Work out the finished part from the listing and answer in its coordinate system (mm). A direction names the side the tool comes from. Round coordinates to 2 decimals unless told otherwise and drop trailing zeros. Write each loop counter-clockwise with the first axis right and the second up, starting at its lowest first coordinate (ties: lowest second). Pieces come first, ordered by that corner, then holes. Notation, with made-up numbers: M 11.5,29.25 L 56.5,29.25 A23 ccw 56.5,59.25 Z; hole C 54,29 d4. An arc over 180 degrees is marked long. Answer in a Markdown table with one row per item.
```python
from build123d import *

# Parameters (mm, degrees)
SKETCH1_R           = 2
SKETCH1_W           = 10
SKETCH1_H           = 28
SKETCH1_W_2         = 12
SKETCH1_H_2         = 48
BOSS_EXTRUDE1_DEPTH = 5
SKETCH1_3_R         = 3.5
BOSS_EXTRUDE2_DEPTH = 8


with BuildPart() as part:
    # Sketch1 → Boss-Extrude1 (new body)
    with BuildSketch(Plane(origin=(0, 0, 0), x_dir=(1, 0, 0), z_dir=(0, 1, 0))):
        with BuildLine():
            Line((0, -9), (0, 9))
            Line((0, 9), (6, 19))
            Line((6, 19), (14, 23.618802154))
            Line((14, 23.618802154), (22, 34))
            Line((22, 34), (22, 40))
            ThreePointArc((22, 40), (23.757359313, 44.242640687), (28, 46))
            Line((28, 46), (36, 46))
            ThreePointArc((36, 46), (40.242640687, 44.242640687), (42, 40))
            Line((42, 40), (42, 34))
            Line((42, 34), (57, 34))
            Line((57, 34), (67, 44))
            Line((67, 44), (87, 44))
            Line((87, 44), (87, 41))
            Line((87, 41), (69, 41))
            Line((69, 41), (69, 37))
            Line((69, 37), (97, 37))
            Line((97, 37), (97, 25))
            Line((97, 25), (87, 25))
            Line((87, 25), (87, 14))
            Line((87, 14), (82, 14))
            Line((82, 14), (82, -14))
            Line((82, -14), (87, -14))
            Line((87, -14), (87, -25))
            Line((87, -25), (97, -25))
            Line((97, -25), (97, -37))
            Line((97, -37), (69, -37))
            Line((69, -37), (69, -41))
            Line((69, -41), (87, -41))
            Line((87, -41), (87, -44))
            Line((87, -44), (67, -44))
            Line((67, -44), (57, -34))
            Line((57, -34), (42, -34))
            Line((42, -34), (42, -40))
            ThreePointArc((42, -40), (40.242640687, -44.242640687), (36, -46))
            Line((36, -46), (28, -46))
            ThreePointArc((28, -46), (23.757359313, -44.242640687), (22, -40))
            Line((22, -40), (22, -34))
            Line((22, -34), (14, -23.618802154))
            Line((14, -23.618802154), (6, -19))
            Line((6, -19), (0, -9))
        make_face()
        with Locations(Location((57, -27, 0), (0, 0, 270))):
            Circle(SKETCH1_R, mode=Mode.SUBTRACT)
        with Locations(Location((7, -10, 0), (0, 0, 270))):
            Circle(SKETCH1_R, mode=Mode.SUBTRACT)
        with Locations(Location((57, 27, 0), (0, 0, 270))):
            Circle(SKETCH1_R, mode=Mode.SUBTRACT)
        with Locations(Location((7, 10, 0), (0, 0, 270))):
            Circle(SKETCH1_R, mode=Mode.SUBTRACT)
        with Locations((66, 0)):
            Rectangle(SKETCH1_W, SKETCH1_H, mode=Mode.SUBTRACT)
        Polygon((14, 19), (23, 24), (23, -24), (14, -19), align=None, mode=Mode.SUBTRACT)
        with Locations((35, 0)):
            Rectangle(SKETCH1_W_2, SKETCH1_H_2, mode=Mode.SUBTRACT)
    extrude(amount=BOSS_EXTRUDE1_DEPTH)

    # Sketch1_3 → Boss-Extrude2 (add)
    with BuildSketch(Plane(origin=(0, 0, 0), x_dir=(1, 0, 0), z_dir=(0, 1, 0))):
        with Locations(Location((32, -40, 0), (0, 0, 270))):
            Circle(SKETCH1_3_R)
        with Locations(Location((32, 40, 0), (0, 0, 270))):
            Circle(SKETCH1_3_R)
    extrude(amount=BOSS_EXTRUDE2_DEPTH)


solid = part.part
```
1. The part is cut by section B-B (z = 17). Determine the outline of the cut face in (x, y).
Calculated:
| item | result |
|---|---|
| outline | M 4.8,0 L 14,0 L 14,5 L 4.8,5 Z; M 23,0 L 29,0 L 29,5 L 23,5 Z; M 41,0 L 87,0 L 87,5 L 41,5 Z |
2. Determine the mould class of faces 1 (the flat face through (84, 2, 14)), 2 (the flat face through (23, 2, 0)), 3 (the flat face through (87, 2, -20)) for opening direction X: released by +X, released by -X, zero draft, split by the parting line, or undercut.
Calculated:
| item | result |
|---|---|
| face 1 | zero draft |
| face 2 | undercut |
| face 3 | released by +X |
3. The part is cut by section A-A (x = 32). Determine the outline of the cut face in (y, z).
Calculated:
| item | result |
|---|---|
| outline | M 0,-46 L 5,-46 L 5,-43.5 L 8,-43.5 L 8,-36.5 L 5,-36.5 L 5,-24 L 0,-24 Z; M 0,24 L 5,24 L 5,36.5 L 8,36.5 L 8,43.5 L 5,43.5 L 5,46 L 0,46 Z |
4. A tool of negligible diameter and unlimited length cuts with its end or side. For faces 4 (the flat face through (42, 2, 37)), 5 (the flat face through (69, 2, 39)), 6 (the flat face through (77, 2, 44)), 7 (the flat face through (77, 2, -44)), 8 (the flat face through (66, 2, 14)), from which of +Z, -Z, +X, -X, +Y, -Y can it reach the whole face along a straight path? Write none if from no direction.
Calculated:
| item | result |
|---|---|
| face 4 | +Z, +Y, -Y |
| face 5 | +X, +Y, -Y |
| face 6 | +Z, +X, +Y, -Y |
| face 7 | -Z, +X, +Y, -Y |
| face 8 | +Y, -Y |
5. Given pin 1 (4 mm diameter, centred on x = 89.5, y = 1.5, fed in from -Z); pin 2 (1.5 mm diameter, centred on x = 60.5, z = -28.5, fed in from +Y); pin 3 (1.5 mm diameter, centred on x = 75, y = 5, fed in from -Z), each flat-ended and moving along its own axis, determine where each tip first touches the part or whether it passes through.
Calculated:
| item | result |
|---|---|
| pin 1 | stops at z = -37 |
| pin 2 | stops at y = 5 |
| pin 3 | stops at z = -44 |
6. The part is cut by section C-C (x = 77.5). Determine the outline of the cut face in (y, z).
Calculated:
| item | result |
|---|---|
| outline | M 0,-44 L 5,-44 L 5,-41 L 0,-41 Z; M 0,-37 L 5,-37 L 5,37 L 0,37 Z; M 0,41 L 5,41 L 5,44 L 0,44 Z |
7. Consider line 1 along X through (y, z) = (4.5, 19); line 2 along X through (y, z) = (4.5, 4); line 3 along X through (y, z) = (1.3, -10). Determine where each line is inside the solid, lowest interval first. Write a range as from..to.
Calculated:
| item | result |
|---|---|
| line 1 | x = 6..14, 23..29, 41..87 |
| line 2 | x = 0..14, 23..29, 41..61, 71..82 |
| line 3 | x = 0.6..5, 9..14, 23..29, 41..61, 71..82 |
8. The part is cut by section D-D (z = -27). Determine the outline of the cut face in (x, y), plus the area to 3 significant figures.
Calculated:
| item | result |
|---|---|
| outline | M 16.61,0 L 55,0 L 55,5 L 16.61,5 Z; M 59,0 L 97,0 L 97,5 L 59,5 Z |
| area | 382 mm² |
